Job drawing, mm, ordinate dimensions from the low corner. One solid piece. Coordinates: 2 decimals unless noted, no trailing zeros. Order: outer loops, then holes, each group sorted by start corner. A loop starts at its lowest first (then second) coordinate and runs counter-clockwise, first axis right, second up. Notation, with made-up numbers: (77, 67.5) -> (116, 67.5) arc R18 cw to (116, 94.5) -> close; hole circle Ø4 at (0.25, 51.25). An arc over 180 degrees is marked (long way). Use CSV: the item, a comma, the result in double quotes. Start each with the question number.
(1) Cut at C-C on x = 26.25. Write the cut outline in (y, z).
(2) Probe L1, parallel to X at y = 1.1, z = 35.75; L2, parallel to Z at x = 26.25, y = 1.9; L3, parallel to Z at x = 19.25, y = 1.1. List the from-to ranges inside material, lowest first.
(3) Cut at D-D on z = 35.75. Write the cut outline in (x, y).
(4) Cut at B-B on y = 1.7. Write the cut outline in (x, z).
(5) Cut at A-A on z = 51.5. Write the cut outline in (x, y), plus the area to 4 significant figures.
(6) Pin check, flat tips, straight feed: pin 1 Ø0.8 at (y, z) = (1.5, 0.5) entering from +X; pin 2 Ø1.2 at (y, z) = (1, 0.5) entering from -X; pin 3 Ø1.5 at (x, y) = (28, 1) entering from +Z; pin 4 Ø2 at (x, z) = (26.25, 35.75) entering from -Y. Stop position of each tip, or through.
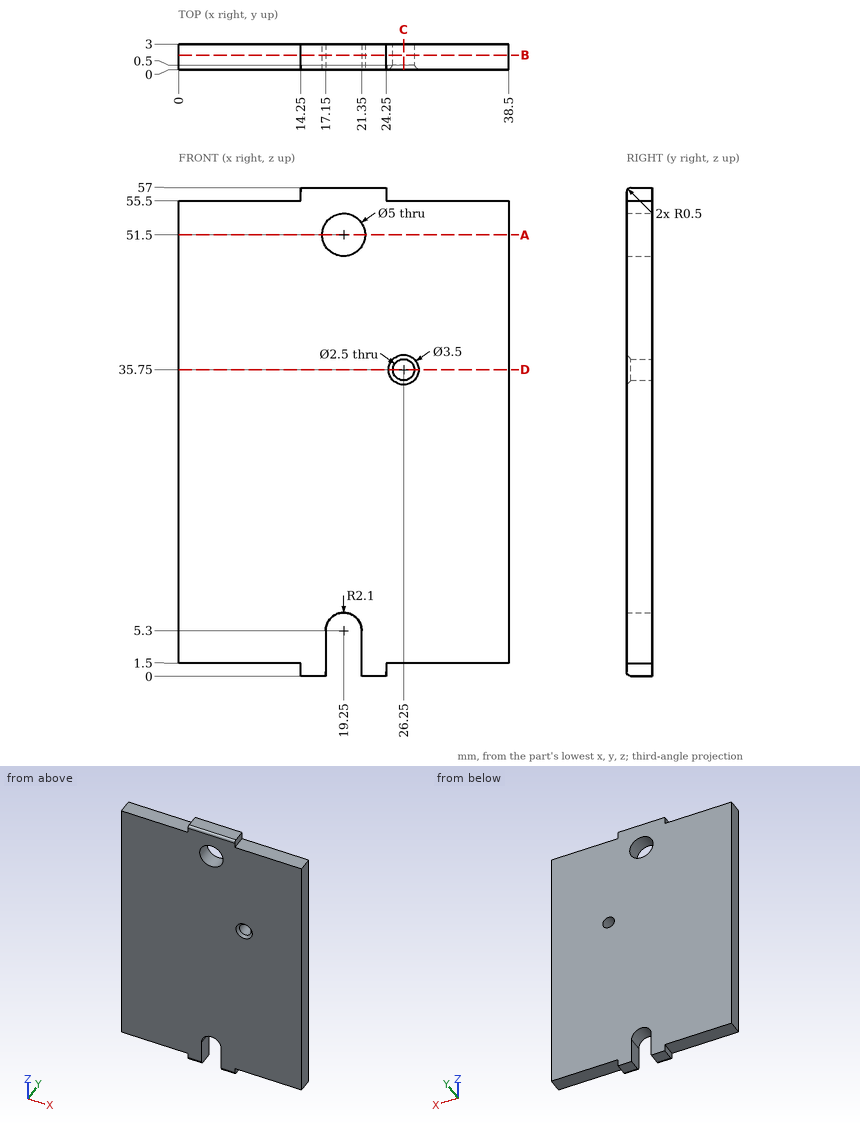
Outcome:
1,outline,"(0, 1.5) -> (3, 1.5) -> (3, 34.5) -> (0.5, 34.5) -> (0, 34) -> close; (0, 37.5) -> (0.5, 37) -> (3, 37) -> (3, 55.5) -> (0, 55.5) -> close"
2,L1,"0 to 25, 27.5 to 38.5"
2,L2,"1.5 to 34.5, 37 to 55.5"
2,L3,"7.4 to 49, 54 to 57"
3,outline,"(0, 0) -> (24.5, 0) -> (25, 0.5) -> (25, 3) -> (0, 3) -> close; (27.5, 0.5) -> (28, 0) -> (38.5, 0) -> (38.5, 3) -> (27.5, 3) -> close"
4,outline,"(0, 1.5) -> (14.25, 1.5) -> (14.25, 0) -> (17.15, 0) -> (17.15, 5.3) arc R2.1 cw to (21.35, 5.3) -> (21.35, 0) -> (24.25, 0) -> (24.25, 1.5) -> (38.5, 1.5) -> (38.5, 55.5) -> (24.25, 55.5) -> (24.25, 57) -> (14.25, 57) -> (14.25, 55.5) -> (0, 55.5) -> close; hole circle Ø5 at (19.25, 51.5); hole circle Ø2.5 at (26.25, 35.75)"
5,outline,"(0, 0) -> (16.75, 0) -> (16.75, 3) -> (0, 3) -> close; (21.75, 0) -> (38.5, 0) -> (38.5, 3) -> (21.75, 3) -> close"
5,area,"100.5 mm2"
6,pin 1,"x = 24.25"
6,pin 2,"x = 14.25"
6,pin 3,"z = 55.5"
6,pin 4,"through"
